Read the model definition and answer for the solid it produces. Units are mm, in the model's axes. Coordinates: 2 decimals unless noted, no trailing zeros. Order: outer loops, then holes, each group sorted by start corner. A loop starts at its lowest first (then second) coordinate and runs counter-clockwise, first axis right, second up. Notation, with made-up numbers: M 79.5,0 L 117.5,0 A28 ccw 117.5,18 Z; hole C 79.5,2.25 d4. An arc over 180 degrees is marked long. Use a Markdown table: item, result. Add a question column.
1) Each of these flat-tipped pins is pushed along its axis until it touches: pin 1 Ø4 at (x, z) = (5, -282.5) entering from +Y; pin 2 Ø5 at (y, z) = (-3, -134) entering from +X; pin 3 Ø2 at (x, z) = (-4.5, -212.5) entering from +Y. Where does it stop, or does it pass through?
2) Find section C-C on z = -109. Write down the section's boundary in (x, y), plus the area to 3 significant figures.
3) Find the intervals of material crossed by probe 1 along Z at (x, y) = (-5.75, -1.5); probe 2 along Y at (x, z) = (-0.75, -294); probe 3 along Y at (x, z) = (5.25, -419), in increasing order. Write a range as [from, to].
from build123d import *

# Parameters (mm, degrees)
SWEEP_1_PROFILE_R   = 8
SKETCH_11_OUTSIDE_W = 118.102
SKETCH_11_OUTSIDE_H = 118.102
SKETCH_11_OUTSIDE_R = 7
CUT_EXTRUDE_1_DEPTH = 20
SKETCH_16_OUTSIDE_W = 118.102
SKETCH_16_OUTSIDE_H = 118.102
SKETCH_16_OUTSIDE_R = 7.5
CUT_EXTRUDE_3_DEPTH = 25
SKETCH_31_W         = 1.1
SKETCH_31_H         = 0.35
SKETCH_12_OUTSIDE_W = 118.102
SKETCH_12_OUTSIDE_H = 118.102
SKETCH_12_OUTSIDE_R = 6
CUT_EXTRUDE_2_DEPTH = 20
SKETCH_3_W          = 1.1
SKETCH_3_H          = 0.25


# Read off the part's stored shape, not the designer's step: M16 机械螺纹 螺柱1
with BuildPart() as part:
    # 扫描1: sweep along a path in 草图1
    with BuildLine(Plane(origin=(0, 0, 0), x_dir=(0, 0, -1), z_dir=(1, 0, 0))) as sweep_1_path:
        Line((0, 0), (500, 0))
    # 扫描1 profile (on start of the path) → 扫描1 (sweep)
    with BuildSketch(Plane(origin=(0, 0, 0), x_dir=(-1, 0, 0), z_dir=(0, 0, -1))):
        Circle(SWEEP_1_PROFILE_R)
    sweep(path=sweep_1_path.line)

    # 草图11 outside → 切除-拉伸1 (cut)
    with BuildSketch(Plane.XY):
        Rectangle(SKETCH_11_OUTSIDE_W, SKETCH_11_OUTSIDE_H)
        Circle(SKETCH_11_OUTSIDE_R, mode=Mode.SUBTRACT)
    extrude(amount=-CUT_EXTRUDE_1_DEPTH, mode=Mode.SUBTRACT)

    # 草图16 outside → 切除-拉伸3 (cut)
    with BuildSketch(Plane.XY.offset(-20)):
        Rectangle(SKETCH_16_OUTSIDE_W, SKETCH_16_OUTSIDE_H)
        Circle(SKETCH_16_OUTSIDE_R, mode=Mode.SUBTRACT)
    extrude(amount=-CUT_EXTRUDE_3_DEPTH, mode=Mode.SUBTRACT)

    # 草图31 → 切除-旋转11 (revolve, cut)
    with BuildSketch(Plane(origin=(100, 0, -20), x_dir=(0, 0, -1), z_dir=(0, 1, 0))):
        with Locations((13.45, 92.675)):
            Rectangle(SKETCH_31_W, SKETCH_31_H)
    revolve(axis=Axis((0, 0, -20), (0, 0, -1)), mode=Mode.SUBTRACT)

    # 草图12 outside → 切除-拉伸2 (cut)
    with BuildSketch(Plane(origin=(0, 0, -500), x_dir=(-1, 0, 0), z_dir=(0, 0, -1))):
        Rectangle(SKETCH_12_OUTSIDE_W, SKETCH_12_OUTSIDE_H)
        Circle(SKETCH_12_OUTSIDE_R, mode=Mode.SUBTRACT)
    extrude(amount=-CUT_EXTRUDE_2_DEPTH, mode=Mode.SUBTRACT)

    # M16 机械螺纹 螺柱1 outline → M16 机械螺纹 螺柱1 (revolve, cut)
    with BuildSketch(Plane.XZ):
        Polygon((8, -45), (6.9175, -45), (8, -46.0825), align=None)
    revolve(axis=Axis((0, 0, 0), (0, 0, 1)), mode=Mode.SUBTRACT)

    # 草图3 → 切除-旋转1 (revolve, cut)
    with BuildSketch(Plane(origin=(-100, 0, -500), x_dir=(0, 0, 1), z_dir=(0, 1, 0))):
        with Locations((4.45, 94.125)):
            Rectangle(SKETCH_3_W, SKETCH_3_H)
    revolve(axis=Axis((0, 0, -500), (0, 0, 1)), mode=Mode.SUBTRACT)


solid = part.part
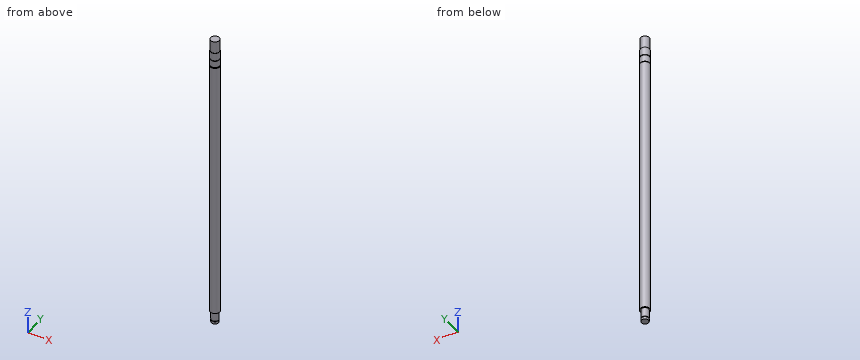
Check result:
| question | item | result |
|---|---|---|
| 1 | pin 1 | stops at y = 7.42 |
| 1 | pin 2 | stops at x = 7.98 |
| 1 | pin 3 | stops at y = 7.19 |
| 2 | outline | C 0,0 d16 |
| 2 | area | 201 mm2 |
| 3 | probe 1 | z = [-500, -496.1], [-495, 0] |
| 3 | probe 2 | y = [-7.96, 7.96] |
| 3 | probe 3 | y = [-6.04, 6.04] |
